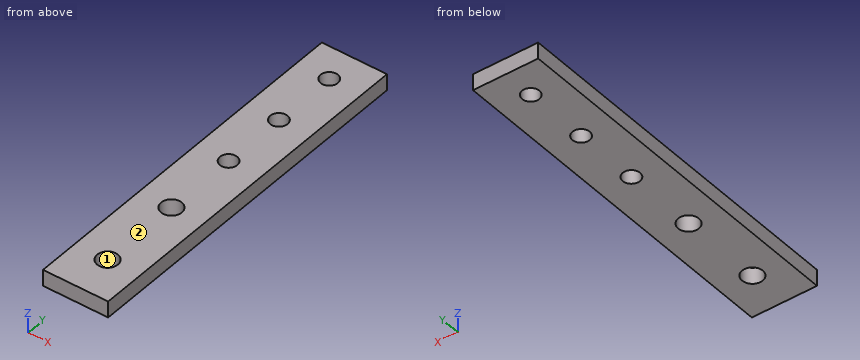
```python
from build123d import *

# Parameters (mm, degrees)
SKETCH1_W                   = 20
SKETCH1_H                   = 110.8
BOSS_EXTRUDE1_DEPTH         = 5
M5_CLEARANCE_HOLE1_D        = 5.3
F_1_4_0_25_DIAMETER_HOLE1_D = 6.35


with BuildPart() as part:
    # Sketch1 → Boss-Extrude1 (new body)
    with BuildSketch(Plane.XY):
        with Locations((6.519823789, 20.433039648)):
            Rectangle(SKETCH1_W, SKETCH1_H)
    extrude(amount=BOSS_EXTRUDE1_DEPTH)

    # M5 Clearance Hole1 (through all)
    with Locations(Plane.XY.offset(5)):
        with Locations((6.519823789, 65.833039648), (6.519823789, 45.833039648), (6.519823789, 25.833039648)):
            Hole(M5_CLEARANCE_HOLE1_D / 2)

    # 1/4 (0.25) Diameter Hole1 (through all)
    with Locations(Plane.XY.offset(5)):
        with Locations((6.519823789, 3.133039648), (6.519823789, -22.266960352)):
            Hole(F_1_4_0_25_DIAMETER_HOLE1_D / 2)


solid = part.part
```
Can you work these out from the model? Positions are in its coordinate system, mm. Face numbers are marked on the shaded views. Coordinates: 2 decimals unless noted, no trailing zeros. Loops run counter-clockwise (first coordinate to the right, second up) from the corner with the lowest first, then second, coordinate; pieces in that order, holes last. Notation, with made-up numbers: (-17, 68.25) - (-6, 68.25) arc R27 cw to (-6, 100.25) - close; hole circle Ø1 at (-5.75, 26). An arc over 180 degrees is marked (long way). Answer as CSV lines item,"result". Start each with the question number.
1) Thinking about a two-plate mould opening in Y: for the marked faces 1 and 2, which applies, pulls with the +Y half, pulls with the -Y half, needs draft (parallel to the pull), parting line crosses it, or undercut?
2) For pin 1 (2 mm diameter, centred on x = 8, y = -11, fed in from -Z), with a flat end and sliding along its axis, tell me the tip position at first contact or that it passes through.
3) Suppose I cut it at A-A (x = 6.25). Please give me the cut outline in (y, z).
4) Suppose I cut it at C-C (z = 3.35). Please give me the cut outline in (x, y) (3 decimals).
5) Suppose I cut it at B-B (y = 24.5). Please give me the cut outline in (x, z).
6) I need wall thicknesses on line 1 (Y direction, x = 6.25, z = 4.6); line 2 (X direction, y = 3, z = 2.9); line 3 (Y direction, x = 5.75, z = 1.35). Which ranges of each line are inside material? Lowest first, please. Write a range as from..to.
Check result:
1,face 1,"undercut"
1,face 2,"needs draft"
2,pin 1,"stops at z = 0"
3,outline,"(-34.97, 0) - (-25.43, 0) - (-25.43, 5) - (-34.97, 5) - close; (-19.1, 0) - (-0.03, 0) - (-0.03, 5) - (-19.1, 5) - close; (6.3, 0) - (23.2, 0) - (23.2, 5) - (6.3, 5) - close; (28.47, 0) - (43.2, 0) - (43.2, 5) - (28.47, 5) - close; (48.47, 0) - (63.2, 0) - (63.2, 5) - (48.47, 5) - close; (68.47, 0) - (75.83, 0) - (75.83, 5) - (68.47, 5) - close"
4,outline,"(-3.48, -34.967) - (16.52, -34.967) - (16.52, 75.833) - (-3.48, 75.833) - close; hole circle Ø6.35 at (6.52, -22.267); hole circle Ø6.35 at (6.52, 3.133); hole circle Ø5.3 at (6.52, 25.833); hole circle Ø5.3 at (6.52, 45.833); hole circle Ø5.3 at (6.52, 65.833)"
5,outline,"(-3.48, 0) - (4.23, 0) - (4.23, 5) - (-3.48, 5) - close; (8.81, 0) - (16.52, 0) - (16.52, 5) - (8.81, 5) - close"
6,line 1,"y = -34.97..-25.43, -19.1..-0.03, 6.3..23.2, 28.47..43.2, 48.47..63.2, 68.47..75.83"
6,line 2,"x = -3.48..3.35, 9.69..16.52"
6,line 3,"y = -34.97..-25.35, -19.19..0.05, 6.21..23.3, 28.37..43.3, 48.37..63.3, 68.37..75.83"
